from build123d import *

# Parameters (mm, degrees)
SKETCH1_W           = 12.7
SKETCH1_H           = 12.7
SKETCH1_R           = 1.1
BOSS_EXTRUDE1_DEPTH = 6.35
SKETCH2_W           = 6.35
SKETCH2_H           = 1
BOSS_EXTRUDE2_DEPTH = 1.68671875
FILLET1_R           = 0.254


with BuildPart() as part:
    # Sketch1 → Boss-Extrude1 (new body)
    with BuildSketch(Plane.XY):
        Rectangle(SKETCH1_W, SKETCH1_H)
        with Locations((-3.81, 0)):
            Circle(SKETCH1_R, mode=Mode.SUBTRACT)
        with Locations((3.81, 0)):
            Circle(SKETCH1_R, mode=Mode.SUBTRACT)
    extrude(amount=BOSS_EXTRUDE1_DEPTH)

    # Sketch2 → Boss-Extrude2 (add, symmetric)
    with BuildSketch(Plane.XY.offset(3.175)):
        with Locations((9.525, 3.0048)):
            Rectangle(SKETCH2_W, SKETCH2_H)
        with Locations((9.525, -3.0048)):
            Rectangle(SKETCH2_W, SKETCH2_H)
    extrude(amount=BOSS_EXTRUDE2_DEPTH, both=True)

    # Fillet1
    fillet1_edges = [part.edges().sort_by_distance(p)[0] for p in [
        (-6.35, 0, 6.35),
        (0, -6.35, 6.35),
        (6.35, 0, 6.35),
        (0, -6.35, 0),
        (-6.35, 0, 0),
        (0, 6.35, 0),
        (6.35, 0, 0),
        (6.35, -6.35, 3.175),
        (-6.35, -6.35, 3.175),
        (-6.35, 6.35, 3.175),
        (6.35, 6.35, 3.175),
        (0, 6.35, 6.35),
    ]]
    fillet(fillet1_edges, radius=FILLET1_R)


solid = part.part
Read the model definition and answer for the solid it produces. Units are mm, in the model's axes. A direction names the side the tool comes from. Coordinates: 2 decimals unless noted, no trailing zeros. Write each loop counter-clockwise with the first axis right and the second up, starting at its lowest first coordinate (ties: lowest second). Pieces come first, ordered by that corner, then holes. Notation, with made-up numbers: (59, 88) -> (113, 88) arc R21 ccw to (113, 119) -> close; hole circle Ø1 at (-19, 48.25). An arc over 180 degrees is marked (long way). Return JSON: item names as keys, results as strings.
(1) The part is cut by section D-D on y = 1.75. Give the vertices of the cut face in (x, z).
Answers below:
{"outline": "(-6.35, 0.25) arc R0.25 ccw to (-6.1, 0) -> (6.1, 0) arc R0.25 ccw to (6.35, 0.25) -> (6.35, 6.1) arc R0.25 ccw to (6.1, 6.35) -> (-6.1, 6.35) arc R0.25 ccw to (-6.35, 6.1) -> close"}
(2) The part is cut by section A-A on x = 3.81. Give the vertices of the cut face in (y, z), then the cut area to 3 significant figures.
Answers below:
{"outline": "(-6.35, 0.25) arc R0.25 ccw to (-6.1, 0) -> (-1.1, 0) -> (-1.1, 6.35) -> (-6.1, 6.35) arc R0.25 ccw to (-6.35, 6.1) -> close; (1.1, 0) -> (6.1, 0) arc R0.25 ccw to (6.35, 0.25) -> (6.35, 6.1) arc R0.25 ccw to (6.1, 6.35) -> (1.1, 6.35) -> close", "area": "66.6 mm^2"}
(3) For a pull along X with two mould halves and no side action, classify faces 6 (the flat face through (12.7, 3, 3)), 7 (the flat face through (0, 0, 0)), 8 (the cylindrical face through (2.71, 0.05, 3.13)) as pulls with the +X half, pulls with the -X half, needs draft (parallel to the pull), parting line crosses it, or undercut.
Answers below:
{"face 6": "pulls with the +X half", "face 7": "needs draft", "face 8": "undercut"}
(4) Consider line 1 along Y through (x, z) = (-3.81, 3); line 2 along Y through (x, z) = (6.5, 2.75); line 3 along X through (y, z) = (-1, 1.5). Determine where each line is inside the solid, lowest interval first. Write a range as from..to.
Answers below:
{"line 1": "-6.35..-1.1, 1.1..6.35", "line 2": "-3.5..-2.5, 2.5..3.5", "line 3": "-6.35..-4.27, -3.35..3.35, 4.27..6.35"}
(5) The part is cut by section B-B on y = 0. Give the vertices of the cut face in (x, z).
Answers below:
{"outline": "(-6.35, 0.25) arc R0.25 ccw to (-6.1, 0) -> (-4.91, 0) -> (-4.91, 6.35) -> (-6.1, 6.35) arc R0.25 ccw to (-6.35, 6.1) -> close; (-2.71, 0) -> (2.71, 0) -> (2.71, 6.35) -> (-2.71, 6.35) -> close; (4.91, 0) -> (6.1, 0) arc R0.25 ccw to (6.35, 0.25) -> (6.35, 6.1) arc R0.25 ccw to (6.1, 6.35) -> (4.91, 6.35) -> close"}
(6) Which of the six approach directions +Z, -Z, +X, -X, +Y, -Y give full straight-line access (tool end or side, diameter ignored) to faces 1 (the flat face through (9, -3, 4.862)), 2 (the flat face through (9, 2.505, 3)), 3 (the flat face through (9, -3.505, 3)), 4 (the flat face through (9, 3.505, 3)), 5 (the flat face through (9, 3, 1.488))?
Answers below:
{"face 1": "+Z, +X, +Y, -Y", "face 2": "+Z, -Z, +X", "face 3": "+Z, -Z, +X, -Y", "face 4": "+Z, -Z, +X, +Y", "face 5": "-Z, +X, +Y, -Y"}
(7) Each of these flat-tipped pins is pushed along its axis until it touches: P1, Ø0.5, axis at x = 9, y = 3, coming from the +Z side; P2, Ø2.5, axis at x = 10.5, z = 3.5, coming from the -Y side; P3, Ø1.8, axis at y = -1, z = 2.5, coming from the +X side. Where does it stop, or does it pass through?
Answers below:
{"P1": "z = 4.86", "P2": "y = -3.5", "P3": "x = 6.35"}
(8) The part is cut by section C-C on z = 4. Give the vertices of the cut face in (x, y), then the cut area to 3 significant figures.
Answers below:
{"outline": "(-6.35, -6.1) arc R0.25 ccw to (-6.1, -6.35) -> (6.1, -6.35) arc R0.25 ccw to (6.35, -6.1) -> (6.35, -3.5) -> (12.7, -3.5) -> (12.7, -2.5) -> (6.35, -2.5) -> (6.35, 2.5) -> (12.7, 2.5) -> (12.7, 3.5) -> (6.35, 3.5) -> (6.35, 6.1) arc R0.25 ccw to (6.1, 6.35) -> (-6.1, 6.35) arc R0.25 ccw to (-6.35, 6.1) -> close; hole circle Ø2.2 at (-3.81, 0); hole circle Ø2.2 at (3.81, 0)", "area": "166 mm^2"}
